For this review, use the dimensioned drawing (mm, ordinates from the lowest corner) and the shaded views. Give positions to 0.01 mm unless a question says otherwise; leave off trailing zeros. Order: outer loops, then holes, each group sorted by start corner. A loop starts at its lowest first (then second) coordinate and runs counter-clockwise, first axis right, second up. Notation, with made-up numbers: (72, 61) -> (121, 61) arc R37 ccw to (121, 99) -> close; hole circle Ø11 at (79.25, -25). An arc over 180 degrees is marked (long way). Return JSON: item names as keys, results as strings.
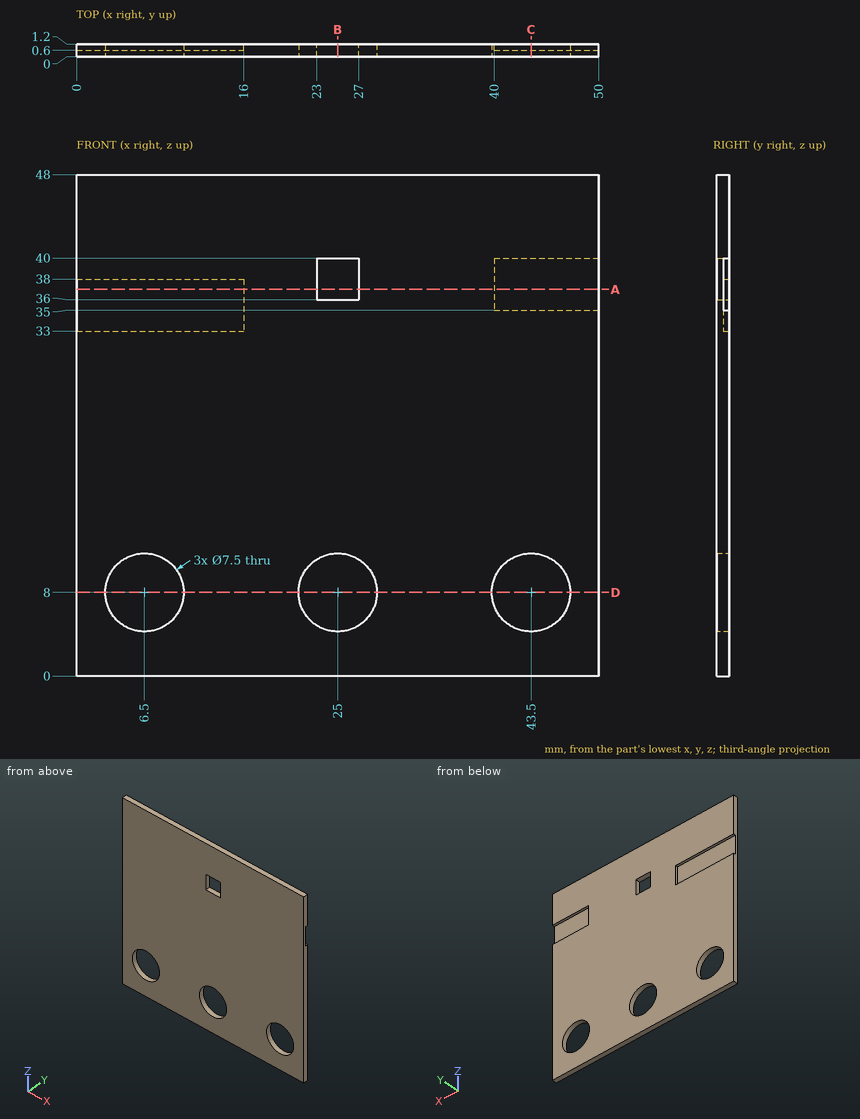
Item 1: Wall thickness on L1, parallel to X at y = 0.3, z = 8; L2, parallel to Z at x = 5, y = 0.45; L3, parallel to X at y = 0.85, z = 11: over which ranges is each line inside the solid? List them lowest first. Write a range as [from, to].
Result set:
{"L1": "x = [0, 2.75], [10.25, 21.25], [28.75, 39.75], [47.25, 50]", "L2": "z = [0, 4.56], [11.44, 48]", "L3": "x = [0, 4.25], [8.75, 22.75], [27.25, 41.25], [45.75, 50]"}
Item 2: Add section D-D (z = 8). Give the boundary of the cut face in (x, y), plus the area to 3 significant figures.
Result set:
{"outline": "(0, 0) -> (2.75, 0) -> (2.75, 1.2) -> (0, 1.2) -> close; (10.25, 0) -> (21.25, 0) -> (21.25, 1.2) -> (10.25, 1.2) -> close; (28.75, 0) -> (39.75, 0) -> (39.75, 1.2) -> (28.75, 1.2) -> close; (47.25, 0) -> (50, 0) -> (50, 1.2) -> (47.25, 1.2) -> close", "area": "33.0 mm^2"}
Item 3: Add section C-C (x = 43.5). Give the boundary of the cut face in (y, z).
Result set:
{"outline": "(0, 0) -> (1.2, 0) -> (1.2, 4.25) -> (0, 4.25) -> close; (0, 11.75) -> (1.2, 11.75) -> (1.2, 35) -> (0.6, 35) -> (0.6, 40) -> (1.2, 40) -> (1.2, 48) -> (0, 48) -> close"}
Item 4: Add section B-B (x = 25). Give the boundary of the cut face in (y, z), plus the area to 3 significant figures.
Result set:
{"outline": "(0, 0) -> (1.2, 0) -> (1.2, 4.25) -> (0, 4.25) -> close; (0, 11.75) -> (1.2, 11.75) -> (1.2, 36) -> (0, 36) -> close; (0, 40) -> (1.2, 40) -> (1.2, 48) -> (0, 48) -> close", "area": "43.8 mm^2"}
Item 5: For pin 1 (2.5 mm diameter, centred on x = 9, z = 35, fed in from +Y), flat-tipped, find the tip position at first contact; note if it passes through.
Result set:
{"pin 1": "stops at y = 0.6"}
Item 6: Add section A-A (z = 37). Give the boundary of the cut face in (x, y), plus the area to 3 significant figures.
Result set:
{"outline": "(0, 0) -> (23, 0) -> (23, 1.2) -> (16, 1.2) -> (16, 0.6) -> (0, 0.6) -> close; (27, 0) -> (50, 0) -> (50, 0.6) -> (40, 0.6) -> (40, 1.2) -> (27, 1.2) -> close", "area": "39.6 mm^2"}
